Read the model definition and answer for the solid it produces. Units are mm, in the model's axes. Face numbers are marked on the shaded views. A direction names the side the tool comes from. Round coordinates to 2 decimals unless told otherwise and drop trailing zeros. Write each loop counter-clockwise with the first axis right and the second up, starting at its lowest first coordinate (ties: lowest second). Pieces come first, ordered by that corner, then holes. Notation, with made-up numbers: (-20.5, 43.25) -> (16.5, 43.25) arc R25 cw to (16.5, 72.25) -> close; hole circle Ø7 at (27.5, -6.75). An arc over 180 degrees is marked (long way). Return JSON: item names as keys, results as strings.
from build123d import *

# Parameters (mm, degrees)
SKETCH_1_W          = 25
SKETCH_1_H          = 30
SKETCH_1_R          = 3.2
EXTRUDE_1_DEPTH     = 4
SKETCH_2_W          = 8
SKETCH_2_H          = 40.4
SKETCH_2_R          = 1.15
EXTRUDE_2_DEPTH     = 6.5
SKETCH_5_R          = 5.2
CUT_EXTRUDE_1_DEPTH = 6.5
SKETCH_6_W          = 8
SKETCH_6_H          = 5.2
EXTRUDE_4_DEPTH     = 4
CUT_EXTRUDE_2_DEPTH = 9
SKETCH_8_W          = 8
SKETCH_8_H          = 2.3
EXTRUDE_5_DEPTH     = 15
FILLET_2_R          = 0.5


with BuildPart() as part:
    # 스케치1 → 보스-돌출1 (new body)
    with BuildSketch(Plane.XY):
        Rectangle(SKETCH_1_W, SKETCH_1_H)
        with Locations((0, 7.5)):
            Circle(SKETCH_1_R, mode=Mode.SUBTRACT)
        with Locations((0, -7.5)):
            Circle(SKETCH_1_R, mode=Mode.SUBTRACT)
    extrude(amount=EXTRUDE_1_DEPTH)

    # 스케치2 → 보스-돌출2 (add)
    with BuildSketch(Plane.XY.offset(4)):
        Rectangle(SKETCH_2_W, SKETCH_2_H)
        Circle(SKETCH_2_R, mode=Mode.SUBTRACT)
        with Locations((0, 15)):
            Circle(SKETCH_2_R, mode=Mode.SUBTRACT)
        with Locations((0, -15)):
            Circle(SKETCH_2_R, mode=Mode.SUBTRACT)
    extrude(amount=EXTRUDE_2_DEPTH)

    # 스케치5 → 컷-돌출1 (cut)
    with BuildSketch(Plane.XY.offset(4)):
        with Locations((0, 7.5)):
            Circle(SKETCH_5_R)
        with Locations((0, -7.5)):
            Circle(SKETCH_5_R)
    extrude(amount=CUT_EXTRUDE_1_DEPTH, mode=Mode.SUBTRACT)

    # 스케치6 → 보스-돌출4 (add)
    with BuildSketch(Plane(origin=(0, 0, 4), x_dir=(-1, 0, 0), z_dir=(0, 0, -1))):
        with Locations((0, 17.6)):
            Rectangle(SKETCH_6_W, SKETCH_6_H)
        with Locations((0, -17.6)):
            Rectangle(SKETCH_6_W, SKETCH_6_H)
    extrude(amount=EXTRUDE_4_DEPTH)

    # 스케치7 → 컷-돌출2 (cut)
    with BuildSketch(Plane(origin=(0, 0, 0), x_dir=(-1, 0, 0), z_dir=(0, 0, -1))):
        Polygon((2.511473671, 15), (1.255736835, 17.175), (-1.255736835, 17.175), (-2.511473671, 15), (-1.255736835, 12.825), (1.255736835, 12.825), align=None)
        Polygon((2.511473671, 0), (1.255736835, 2.175), (-1.255736835, 2.175), (-2.511473671, 0), (-1.255736835, -2.175), (1.255736835, -2.175), align=None)
        Polygon((2.511473671, -15), (1.255736835, -12.825), (-1.255736835, -12.825), (-2.511473671, -15), (-1.255736835, -17.175), (1.255736835, -17.175), align=None)
    extrude(amount=-CUT_EXTRUDE_2_DEPTH, mode=Mode.SUBTRACT)

    # 스케치8 → 보스-돌출5 (add)
    with BuildSketch(Plane(origin=(0, 0, 0), x_dir=(-1, 0, 0), z_dir=(0, 0, -1))):
        with Locations((0, 21.35)):
            Rectangle(SKETCH_8_W, SKETCH_8_H)
        with Locations((0, -21.35)):
            Rectangle(SKETCH_8_W, SKETCH_8_H)
    extrude(amount=-EXTRUDE_5_DEPTH)

    # 필렛2
    fillet_2_edges = [part.edges().sort_by_distance(p)[0] for p in [
        (4, -15, 2),
        (-4, -15, 2),
        (-4, 22.5, 7.5),
        (0, 22.5, 15),
        (4, 22.5, 7.5),
        (0, -22.5, 15),
        (-4, -22.5, 7.5),
        (4, -22.5, 7.5),
        (-4, 4.177350455, 7.25),
        (-4, 10.822649545, 7.25),
        (4, 10.822649545, 7.25),
        (4, 4.177350455, 7.25),
        (-12.5, 15, 2),
        (12.5, 15, 2),
        (-4, -10.822649545, 7.25),
        (-4, -4.177350455, 7.25),
        (12.5, -15, 2),
        (4, -4.177350455, 7.25),
        (4, -10.822649545, 7.25),
        (-12.5, -15, 2),
        (-4, 15, 2),
        (4, 15, 2),
    ]]
    fillet(fillet_2_edges, radius=FILLET_2_R)


solid = part.part
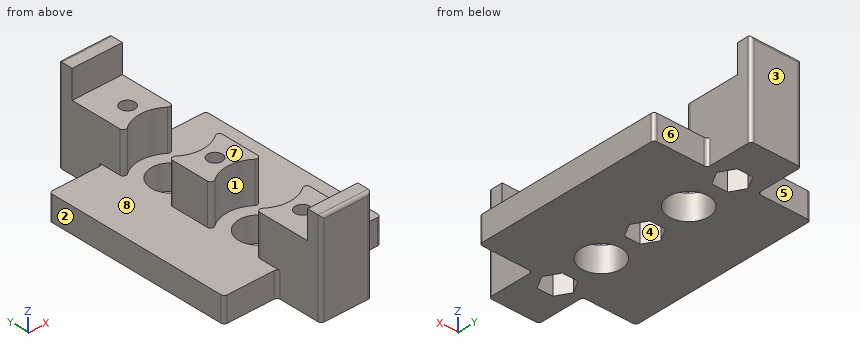
Item 1: For a pull along Y with two mould halves and no side action, classify the marked faces 1, 2, 3 and 4 as released by +Y, released by -Y, zero draft, split by the parting line, or undercut.
Worked answers:
{"face 1": "undercut", "face 2": "zero draft", "face 3": "released by +Y", "face 4": "undercut"}
Item 2: Straight lines are drawn through the part: L1, parallel to Y at x = 0, z = 1.3 (3 decimals); L2, parallel to X at y = -15, z = 7.5; L3, parallel to Y at x = 0, z = 10.15. For each, find the intervals that lie inside material, in ascending order. Write a range as [from, to].
Worked answers:
{"L1": "y = [-22.5, -17.175], [-12.825, -10.7], [-4.3, -2.175], [2.175, 4.3], [10.7, 12.825], [17.175, 22.5]", "L2": "x = [-4, -2.51], [2.51, 4]", "L3": "y = [-22.5, -16.15], [-13.85, -12.7], [-2.3, -1.15], [1.15, 2.3], [12.7, 13.85], [16.15, 22.5]"}
Item 3: A tool of negligible diameter and unlimited length cuts with its end or side. For the marked faces 5, 6, 7 and 8, from which of +Z, -Z, +X, -X, +Y, -Y can it reach the whole face along a straight path? Write none if from no direction.
Worked answers:
{"face 5": "+Z, -Z, -X, +Y", "face 6": "+Z, -Z, +X, +Y", "face 7": "+Z, +X, -X", "face 8": "+Z"}
Item 4: Section D-D (y = -0.5) is taken. Give the vertices of the cut face in (x, z).
Worked answers:
{"outline": "(-12.5, 0) -> (-2.22, 0) -> (-2.22, 9) -> (-1.04, 9) -> (-1.04, 10.5) -> (-4, 10.5) -> (-4, 4) -> (-12.5, 4) -> close; (1.04, 9) -> (2.22, 9) -> (2.22, 0) -> (12.5, 0) -> (12.5, 4) -> (4, 4) -> (4, 10.5) -> (1.04, 10.5) -> close"}
Item 5: Section C-C (x = 0) is taken. State how many separate pieces and enclosed holes the cut face has, then the cut area to 3 significant figures.
Worked answers:
{"separate pieces": "6", "enclosed holes": "0", "area": "179 mm2"}
Item 6: Section A-A (z = 10) is taken. Give the vertices of the cut face in (x, y), then the cut area to 3 significant figures.
Worked answers:
{"outline": "(-4, -22) arc R0.5 ccw to (-3.5, -22.5) -> (3.5, -22.5) arc R0.5 ccw to (4, -22) -> (4, -12) arc R0.5 ccw to (3.19, -11.6) arc R5.2 cw to (-3.19, -11.6) arc R0.5 ccw to (-4, -12) -> close; (-4, -3) arc R0.5 ccw to (-3.19, -3.4) arc R5.2 cw to (3.19, -3.4) arc R0.5 ccw to (4, -3) -> (4, 3) arc R0.5 ccw to (3.19, 3.4) arc R5.2 cw to (-3.19, 3.4) arc R0.5 ccw to (-4, 3) -> close; (-4, 12) arc R0.5 ccw to (-3.19, 11.6) arc R5.2 cw to (3.19, 11.6) arc R0.5 ccw to (4, 12) -> (4, 22) arc R0.5 ccw to (3.5, 22.5) -> (-3.5, 22.5) arc R0.5 ccw to (-4, 22) -> close; hole circle Ø2.3 at (0, -15); hole circle Ø2.3 at (0, 0); hole circle Ø2.3 at (0, 15)", "area": "197 mm2"}
Item 7: Flat-ended cylindrical pins translate along their axes: pin 1 (3 mm diameter, centred on y = -1.5, z = 9.5, fed in from -X); pin 2 (3 mm diameter, centred on x = 0, y = 15, fed in from +Z); pin 3 (4.5 mm diameter, centred on x = 6.5, z = 2.5, fed in from +Y). Find the tip coordinate at first contact, or state that the pin passes through.
Worked answers:
{"pin 1": "stops at x = -4", "pin 2": "stops at z = 10.5", "pin 3": "stops at y = 15.07"}
Item 8: Section B-B (y = -7.5) is taken. Give the vertices of the cut face in (x, z).
Worked answers:
{"outline": "(-12.5, 0) -> (-3.2, 0) -> (-3.2, 4) -> (-12.5, 4) -> close; (3.2, 0) -> (12.5, 0) -> (12.5, 4) -> (3.2, 4) -> close"}
